Could you check a few things on this model? Use its own coordinates, in mm. A direction names the side the tool comes from. Coordinates: 2 decimals unless noted, no trailing zeros. Write each loop counter-clockwise with the first axis right and the second up, starting at its lowest first coordinate (ties: lowest second). Pieces come first, ordered by that corner, then holes.
```python
from build123d import *

# Parameters (mm, degrees)
F0_R     = 7.588
F0_R_2   = 1.105
F1_DEPTH = 1.32


with BuildPart() as f1:
    # F0 (on Top) → F1 (new body)
    with BuildSketch(Plane.XY):
        Circle(F0_R)
        with BuildLine():
            ThreePointArc((-0.075923, -1.978544), (0.99, -1.71473), (1.751431, -0.923521))
            ThreePointArc((1.751431, -0.923521), (2.798444, -0.599465), (3.1225, -1.646479))
            ThreePointArc((3.1225, -1.646479), (1.765, -3.05707), (-0.135357, -3.527404))
            ThreePointArc((-0.135357, -3.527404), (-0.88007, -2.723257), (-0.075923, -1.978544))
        make_face(mode=Mode.SUBTRACT)
        with BuildLine():
            ThreePointArc((-2.987143, 1.880925), (-1.918374, 2.123791), (-1.675508, 1.055023))
            ThreePointArc((-1.675508, 1.055023), (-1.98, 0), (-1.675508, -1.055023))
            ThreePointArc((-1.675508, -1.055023), (-1.918374, -2.123791), (-2.987143, -1.880925))
            ThreePointArc((-2.987143, -1.880925), (-3.53, 0), (-2.987143, 1.880925))
        make_face(mode=Mode.SUBTRACT)
        Circle(F0_R_2, mode=Mode.SUBTRACT)
        with BuildLine():
            ThreePointArc((3.1225, 1.646479), (2.798444, 0.599465), (1.751431, 0.923521))
            ThreePointArc((1.751431, 0.923521), (0.99, 1.71473), (-0.075923, 1.978544))
            ThreePointArc((-0.075923, 1.978544), (-0.88007, 2.723257), (-0.135357, 3.527404))
            ThreePointArc((-0.135357, 3.527404), (1.765, 3.05707), (3.1225, 1.646479))
        make_face(mode=Mode.SUBTRACT)
    extrude(amount=F1_DEPTH)


solid = f1.part
```
1. On a 3-axis mill with a long thin cutter (end or side, diameter ignored), from which of +Z, -Z, +X, -X, +Y, -Y can I reach the whole of each face in a straight line? I mean faces 4 (the face through (2, 0, 1.32)), 5 (the face through (1.789, -3.043, 0.651)). Say none if no direction works.
Verdict:
face 4: +Z, +X, -X, +Y, -Y
face 5: +Z, -Z
2. I want a section at B-B on x = 2.5. Please give me the cut outline in (y, z).
Verdict:
outline: (-7.16, 0) - (-2.49, 0) - (-2.49, 1.32) - (-7.16, 1.32) - close; (-0.51, 0) - (0.51, 0) - (0.51, 1.32) - (-0.51, 1.32) - close; (2.49, 0) - (7.16, 0) - (7.16, 1.32) - (2.49, 1.32) - close
3. I want a section at C-C on z = 0.5. Give the number of separate pieces and of enclosed holes in the cut face, plus the area to 3 significant figures.
Verdict:
separate pieces: 1
enclosed holes: 4
area: 157 mm2
4. I want a section at A-A on y = 0. Please give me the cut outline in (x, z) (3 decimals).
Verdict:
outline: (-7.588, 0) - (-3.53, 0) - (-3.53, 1.32) - (-7.588, 1.32) - close; (-1.98, 0) - (-1.105, 0) - (-1.105, 1.32) - (-1.98, 1.32) - close; (1.105, 0) - (7.588, 0) - (7.588, 1.32) - (1.105, 1.32) - close
5. I want a section at D-D on x = 6.75. Please give me the cut outline in (y, z), plus the area to 3 significant figures.
Verdict:
outline: (-3.47, 0) - (3.47, 0) - (3.47, 1.32) - (-3.47, 1.32) - close
area: 9.15 mm2
6. For pin 1 (1.3 mm diameter, centred on x = 0, y = 0, fed in from -Z), with a flat end and sliding along its axis, tell me the tip position at first contact or that it passes through.
Verdict:
pin 1: passes through
7. Please list where these lines run through material, in increasing order: line 1 along Y through (x, z) = (0, 0.6) (3 decimals); line 2 along Y through (x, z) = (2, 1.05); line 3 along Y through (x, z) = (1, 0.3).
Verdict:
line 1: y = -7.588 to -3.53, -1.98 to -1.105, 1.105 to 1.98, 3.53 to 7.588
line 2: y = -7.32 to -2.91, -0.64 to 0.64, 2.91 to 7.32
line 3: y = -7.52 to -3.39, -1.71 to -0.47, 0.47 to 1.71, 3.39 to 7.52
8. If we mould it in two halves opening along X, with no side actions, what happens to faces 1 (the face through (2, 0, 0)), 2 (the face through (2.8, 0.6, 0.7)), 3 (the face through (-1.64, -7.41, 0.65))? For each: pulls with the +X half, pulls with the -X half, needs draft (parallel to the pull), parting line crosses it, or undercut.
Verdict:
face 1: needs draft
face 2: undercut
face 3: parting line crosses it
